from build123d import *

# Parameters (mm, degrees)
F0_W      = 40.7
F0_H      = 100
F1_DEPTH  = 1
F2_W      = 40.7
F2_H      = 100
F2_W_2    = 6
F2_H_2    = 88
F3_DEPTH  = 3.9
F4_W      = 40.7
F4_H      = 1.85
F5_DEPTH  = 5
F6_R      = 1.6
F7_DEPTH  = 1.851
F8_W      = 20
F8_H      = 2
F9_DEPTH  = 6
F10_W     = 20
F10_H     = 2
F11_DEPTH = 6


# Not quite as in the source:
# - a pattern or mirror of a feature is missing from the dataset's text; its kind, count and spacing are read off the source's solid


with BuildPart() as f1:
    # F0 (on Top) → F1 (new body)
    with BuildSketch(Plane.XY):
        Rectangle(F0_W, F0_H)
    extrude(amount=-F1_DEPTH)

    # F2 (on Top) → F3 (join)
    with BuildSketch(Plane.XY):
        Rectangle(F2_W, F2_H)
        Polygon((-14.35, -44), (-14.35, 44), (-3, 44), (3, 44), (14.35, 44), (14.35, -44), (3, -44), (-3, -44), align=None, mode=Mode.SUBTRACT)
        Rectangle(F2_W_2, F2_H_2)
    extrude(amount=F3_DEPTH)

    # F4 (on face) → F5 (join)
    with BuildSketch(Plane.XZ.offset(50)):
        with Locations((0, 2.975)):
            Rectangle(F4_W, F4_H)
    f5 = extrude(amount=F5_DEPTH)

    # F5_copies: F5 across plane
    add(f5.mirror(Plane.ZX))

    # F6 (on face) → F7 (cut, through all)
    with BuildSketch(Plane(origin=(0, 0, 2.05), x_dir=(1, 0, 0), z_dir=(0, 0, -1))):
        with Locations((-15, 52.5)):
            Circle(F6_R)
        with Locations((15, 52.5)):
            Circle(F6_R)
        with Locations((-15, -52.5)):
            Circle(F6_R)
        with Locations((15, -52.5)):
            Circle(F6_R)
    extrude(amount=-F7_DEPTH, mode=Mode.SUBTRACT)

    # F8 (on face) → F9 (cut, through all)
    with BuildSketch(Plane(origin=(-20.35, 0, 0), x_dir=(0, -1, 0), z_dir=(-1, 0, 0))):
        with Locations((-30, 1.45)):
            Rectangle(F8_W, F8_H)
        with Locations((30, 1.45)):
            Rectangle(F8_W, F8_H)
    extrude(amount=-F9_DEPTH, mode=Mode.SUBTRACT)

    # F10 (on face) → F11 (cut, through all)
    with BuildSketch(Plane.YZ.offset(20.35)):
        with Locations((-30, 1.45)):
            Rectangle(F10_W, F10_H)
        with Locations((30, 1.45)):
            Rectangle(F10_W, F10_H)
    extrude(amount=-F11_DEPTH, mode=Mode.SUBTRACT)


solid = f1.part
Could you check a few things on this model? Use its own coordinates, in mm. A direction names the side the tool comes from. Give positions to 0.01 mm unless a question says otherwise; leave off trailing zeros. Loops run counter-clockwise (first coordinate to the right, second up) from the corner with the lowest first, then second, coordinate; pieces in that order, holes last. Notation, with made-up numbers: M 65.25,6 L 119.25,6 A32 ccw 119.25,36 Z; hole C 57,26.5 d6. An arc over 180 degrees is marked long. Answer as a JSON object with one key per item and string values.
Q1. For faces 1 (the flat face through (-14.35, -1, 2)), 2 (the flat face through (-17, -40, 1)), 3 (the flat face through (17, 40, 1)), which set-ups out of +Z, -Z, +X, -X, +Y, -Y let a thin tool reach every point of the face, with its end or its side?
Values found:
{"face 1": "+Z", "face 2": "-X", "face 3": "+X"}
Q2. Suppose I cut it at D-D, the plane y = 42.5. List the corners of the cut face in (x, z) for me, plus the area to 3 significant figures.
Values found:
{"outline": "M -20.35,-1 L 20.35,-1 L 20.35,3.9 L 14.35,3.9 L 14.35,0 L 3,0 L 3,3.9 L -3,3.9 L -3,0 L -14.35,0 L -14.35,3.9 L -20.35,3.9 Z", "area": "111 mm²"}
Q3. Suppose I cut it at A-A, the plane y = 30.5. List the corners of the cut face in (x, z) for me.
Values found:
{"outline": "M -20.35,-1 L 20.35,-1 L 20.35,0.45 L 14.35,0.45 L 14.35,0 L 3,0 L 3,3.9 L -3,3.9 L -3,0 L -14.35,0 L -14.35,0.45 L -20.35,0.45 Z; M -20.35,2.45 L -14.35,2.45 L -14.35,3.9 L -20.35,3.9 Z; M 14.35,2.45 L 20.35,2.45 L 20.35,3.9 L 14.35,3.9 Z"}
Q4. For P1, Ø5.5, axis at x = 8.5, y = -1.5, coming from the +Z side; P2, Ø1, axis at x = 16.5, z = 1.5, coming from the -Y side, each with a flat end and sliding along its axis, tell me the tip position at first contact or that it passes through.
Values found:
{"P1": "stops at z = 0", "P2": "stops at y = -50"}
Q5. If I drill on probe 1 along X at (y, z) = (52.5, 3.2); probe 2 along X at (y, z) = (0, 0.25); probe 3 along Y at (x, z) = (15, 1.05), over which ranges is the centre line in solid material (lowest first)? Write a range as [from, to].
Values found:
{"probe 1": "x = [-20.35, -16.6], [-13.4, 13.4], [16.6, 20.35]", "probe 2": "x = [-20.35, -14.35], [-3, 3], [14.35, 20.35]", "probe 3": "y = [-50, -40], [-20, 20], [40, 50]"}
Q6. If we mould it in two halves opening along Y, with no side actions, what happens to faces 4 (the flat face through (0, -50, 1)), 5 (the flat face through (-17, 30, 0.45)), 6 (the flat face through (20.35, -1, 1))? For each: pulls with the +Y half, pulls with the -Y half, needs draft (parallel to the pull), parting line crosses it, or undercut.
Values found:
{"face 4": "pulls with the -Y half", "face 5": "undercut", "face 6": "needs draft"}
Q7. Suppose I cut it at C-C, the plane y = -52.5. List the corners of the cut face in (x, z) for me, plus the area to 3 significant figures.
Values found:
{"outline": "M -20.35,2.05 L -16.6,2.05 L -16.6,3.9 L -20.35,3.9 Z; M -13.4,2.05 L 13.4,2.05 L 13.4,3.9 L -13.4,3.9 Z; M 16.6,2.05 L 20.35,2.05 L 20.35,3.9 L 16.6,3.9 Z", "area": "63.5 mm²"}
Q8. Suppose I cut it at B-B, the plane x = 7.5. List the corners of the cut face in (y, z) for me.
Values found:
{"outline": "M -55,2.05 L -50,2.05 L -50,-1 L 50,-1 L 50,2.05 L 55,2.05 L 55,3.9 L 44,3.9 L 44,0 L -44,0 L -44,3.9 L -55,3.9 Z"}
